For this review, take the finished solid that the model builds, in its own axes (mm). A direction names the side the tool comes from. Coordinates: 2 decimals unless noted, no trailing zeros. Loops run counter-clockwise (first coordinate to the right, second up) from the corner with the lowest first, then second, coordinate; pieces in that order, holes last. Notation, with made-up numbers: M 30.25,-38.5 L 64.25,-38.5 A25 cw 64.25,-20.5 Z; hole C -3.75,20.5 d10. An arc over 180 degrees is marked long. Answer as a JSON object with one key per item and string values. Group by question number.
Item 1: Add section A-A (x = 75). State the section outline as (y, z) points.
Item 2: Add section B-B (x = -81). State the section outline as (y, z) points.
Item 3: Wall thickness on L1, parallel to Y at x = 97.5, z = 4.35; L2, parallel to Y at x = 13.5, z = 4.9; L3, parallel to X at y = -73, z = 4.2: over which ranges is each line inside the solid? List them lowest first. Write a range as from..to.
Item 4: Insertion check: pin 1 (1.8 mm diameter, centred on x = 103.5, z = 2.5, fed in from -Y); pin 2 (3 mm diameter, centred on x = 171.5, z = 3, fed in from -Y); pin 3 (1.8 mm diameter, centred on x = -172, z = 4, fed in from +Y). Each pin has a flat end and moves straight along its axis. Give the tip position at first contact, or say it passes through.
Item 5: Mouldability with a two-part tool opening along X and no side actions: class faces 3 (the face through (3, -85, 0)), 4 (the face through (88.97, -78.69, 2.96)) as +X half, -X half, draft (parallel to the pull), parting line (faces both ways), or undercut.
Item 6: Add section C-C (z = 4.7). Count the separate pieces of the cut face and the enclosed holes in it, then the cut area to 3 significant figures.
Item 7: Tool access review of faces 1 (the face through (3, -85, 6)), 2 (the face through (-125.17, -78.85, 2.96)): name each direction out of +Z, -Z, +X, -X, +Y, -Y from which nothing blocks a thin tool from reaching the whole face with its end or side.
from build123d import *

# Parameters (mm, degrees)
SKETCH_1_R      = 1.55
SKETCH_1_R_2    = 7.9
SKETCH_1_R_3    = 1.500000002
SKETCH_1_R_4    = 1.500000001
SKETCH_1_R_5    = 1.5
SKETCH_1_R_6    = 1.25
SKETCH_1_W      = 6
SKETCH_1_H      = 10
SKETCH_1_W_2    = 10
SKETCH_1_H_2    = 6
EXTRUDE_1_DEPTH = 6


with BuildPart() as part:
    # Эскиз1 → Бобышка-Вытянуть1 (new body)
    with BuildSketch(Plane.XY):
        with BuildLine():
            Line((146.728571026, 193.302051095), (172.76481778, 193.302051095))
            ThreePointArc((172.76481778, 193.302051095), (177.038597027, 191.56796477), (178.819099243, 187.313313634))
            Line((178.819099243, 187.313313634), (178.819099243, -193.997982862))
            ThreePointArc((178.819099243, -193.997982862), (177.042504932, -198.259771734), (172.764817781, -199.997737318))
            Line((172.764817781, -199.997737318), (145.728432875, -199.997737318))
            ThreePointArc((145.728432875, -199.997737318), (142.13617765, -199.201353507), (139.217055109, -196.961432))
            Line((139.217055109, -196.961432), (136.921229056, -193.941778905))
            ThreePointArc((136.921229056, -193.941778905), (134.002106514, -191.701857397), (130.409851289, -190.905473587))
            Line((130.409851289, -190.905473587), (-129.880215727, -190.905473587))
            ThreePointArc((-129.880215727, -190.905473587), (-133.472470952, -191.701857397), (-136.391593494, -193.941778905))
            Line((-136.391593494, -193.941778905), (-138.687419547, -196.961432))
            ThreePointArc((-138.687419547, -196.961432), (-141.606542089, -199.201353507), (-145.198797314, -199.997737318))
            Line((-145.198797314, -199.997737318), (-172.235182219, -199.997737318))
            ThreePointArc((-172.235182219, -199.997737318), (-175.957867453, -198.836968562), (-178.180900757, -195.633237551))
            Line((-178.180900757, -195.633237551), (-178.180900757, 187.302262682))
            ThreePointArc((-178.180900757, 187.302262682), (-176.423541444, 191.54490337), (-172.180900757, 193.302262682))
            Line((-172.180900757, 193.302262682), (-146.198797315, 193.302262682))
            ThreePointArc((-146.198797315, 193.302262682), (-142.60654209, 194.098646493), (-139.687419548, 196.338568))
            Line((-139.687419548, 196.338568), (-136.391593495, 200.265957365))
            ThreePointArc((-136.391593495, 200.265957365), (-133.472470953, 202.505878872), (-129.880215728, 203.302262682))
            Line((-129.880215728, 203.302262682), (130.409851288, 203.302262682))
            ThreePointArc((130.409851288, 203.302262682), (134.002106513, 202.505878872), (136.921229055, 200.265957365))
            Line((136.921229055, 200.265957365), (140.217104458, 196.338462244))
            ThreePointArc((140.217104458, 196.338462244), (143.136253197, 194.098464098), (146.728571026, 193.302051095))
        make_face()
        with Locations((108.319099243, 165.602262682)):
            Circle(SKETCH_1_R, mode=Mode.SUBTRACT)
        with Locations((108.319099243, 175.302262682)):
            Circle(SKETCH_1_R, mode=Mode.SUBTRACT)
        with Locations((131.519099243, 180.302262682)):
            Circle(SKETCH_1_R_2, mode=Mode.SUBTRACT)
        with Locations((-151.980900757, 180.302262682)):
            Circle(SKETCH_1_R_2, mode=Mode.SUBTRACT)
        with Locations((-171.180900757, 150.902262682)):
            Circle(SKETCH_1_R_3, mode=Mode.SUBTRACT)
        with Locations((-171.180900757, 16.742262682)):
            Circle(SKETCH_1_R_4, mode=Mode.SUBTRACT)
        with Locations((171.819099243, 150.902051095)):
            Circle(SKETCH_1_R_4, mode=Mode.SUBTRACT)
        with Locations((126.459099243, 196.302262682)):
            Circle(SKETCH_1_R_5, mode=Mode.SUBTRACT)
        with Locations((-125.820900757, 196.302262682)):
            Circle(SKETCH_1_R_5, mode=Mode.SUBTRACT)
        with Locations((0.319099243, 196.302262682)):
            Circle(SKETCH_1_R_5, mode=Mode.SUBTRACT)
        with Locations((-119.870900757, -136.997737318)):
            Circle(SKETCH_1_R_5, mode=Mode.SUBTRACT)
        with Locations((-171.180900757, -114.967737318)):
            Circle(SKETCH_1_R_5, mode=Mode.SUBTRACT)
        with Locations((0.319099243, -136.997737318)):
            Circle(SKETCH_1_R_5, mode=Mode.SUBTRACT)
        with Locations((120.509099243, -136.997737318)):
            Circle(SKETCH_1_R_5, mode=Mode.SUBTRACT)
        with Locations((171.819099243, -114.967948905)):
            Circle(SKETCH_1_R_5, mode=Mode.SUBTRACT)
        with Locations((171.819099244, 16.742051095)):
            Circle(SKETCH_1_R_5, mode=Mode.SUBTRACT)
        with Locations((-139.980900757, 180.302262682)):
            Circle(SKETCH_1_R_6, mode=Mode.SUBTRACT)
        with Locations((-163.980900757, 180.302262682)):
            Circle(SKETCH_1_R_6, mode=Mode.SUBTRACT)
        with Locations((119.519099243, 180.302262682)):
            Circle(SKETCH_1_R_6, mode=Mode.SUBTRACT)
        with Locations((143.519099243, 180.302262682)):
            Circle(SKETCH_1_R_6, mode=Mode.SUBTRACT)
        with BuildLine():
            Line((133.65547985, 83.46981119), (133.65547985, 87.96981119))
            ThreePointArc((133.65547985, 87.96981119), (132.05547985, 89.56981119), (130.45547985, 87.96981119))
            Line((130.45547985, 87.96981119), (130.45547985, 83.46981119))
            ThreePointArc((130.45547985, 83.46981119), (132.05547985, 81.86981119), (133.65547985, 83.46981119))
        make_face(mode=Mode.SUBTRACT)
        with BuildLine():
            Line((133.65547985, 118.96981119), (133.65547985, 114.46981119))
            ThreePointArc((133.65547985, 114.46981119), (132.05547985, 112.86981119), (130.45547985, 114.46981119))
            Line((130.45547985, 114.46981119), (130.45547985, 118.96981119))
            ThreePointArc((130.45547985, 118.96981119), (132.05547985, 120.56981119), (133.65547985, 118.96981119))
        make_face(mode=Mode.SUBTRACT)
        with BuildLine():
            Line((158.55547985, 98.96981119), (158.55547985, 103.46981119))
            ThreePointArc((158.55547985, 103.46981119), (147.55547985, 114.46981119), (136.55547985, 103.46981119))
            Line((136.55547985, 103.46981119), (136.55547985, 98.96981119))
            ThreePointArc((136.55547985, 98.96981119), (147.55547985, 87.96981119), (158.55547985, 98.96981119))
        make_face(mode=Mode.SUBTRACT)
        with BuildLine():
            Line((161.45547985, 118.96981119), (161.45547985, 114.46981119))
            ThreePointArc((161.45547985, 114.46981119), (163.05547985, 112.86981119), (164.65547985, 114.46981119))
            Line((164.65547985, 114.46981119), (164.65547985, 118.96981119))
            ThreePointArc((164.65547985, 118.96981119), (163.05547985, 120.56981119), (161.45547985, 118.96981119))
        make_face(mode=Mode.SUBTRACT)
        with BuildLine():
            Line((161.45547985, 83.46981119), (161.45547985, 87.96981119))
            ThreePointArc((161.45547985, 87.96981119), (163.05547985, 89.56981119), (164.65547985, 87.96981119))
            Line((164.65547985, 87.96981119), (164.65547985, 83.46981119))
            ThreePointArc((164.65547985, 83.46981119), (163.05547985, 81.86981119), (161.45547985, 83.46981119))
        make_face(mode=Mode.SUBTRACT)
        with Locations((-171.180900756, 41.742262682)):
            Rectangle(SKETCH_1_W, SKETCH_1_H, mode=Mode.SUBTRACT)
        with Locations((94.109099243, -136.997737318)):
            Rectangle(SKETCH_1_W_2, SKETCH_1_H_2, mode=Mode.SUBTRACT)
        with Locations((146.909099243, -136.997737318)):
            Rectangle(SKETCH_1_W_2, SKETCH_1_H_2, mode=Mode.SUBTRACT)
        with Locations((-24.670900757, 196.302262682)):
            Rectangle(SKETCH_1_W_2, SKETCH_1_H_2, mode=Mode.SUBTRACT)
        with Locations((25.309099243, 196.302262682)):
            Rectangle(SKETCH_1_W_2, SKETCH_1_H_2, mode=Mode.SUBTRACT)
        with Locations((-146.270900757, -136.997737318)):
            Rectangle(SKETCH_1_W_2, SKETCH_1_H_2, mode=Mode.SUBTRACT)
        with Locations((-93.470900757, -136.997737318)):
            Rectangle(SKETCH_1_W_2, SKETCH_1_H_2, mode=Mode.SUBTRACT)
        with Locations((-25.470900757, -136.997737318)):
            Rectangle(SKETCH_1_W_2, SKETCH_1_H_2, mode=Mode.SUBTRACT)
        with Locations((26.109099243, -136.997737318)):
            Rectangle(SKETCH_1_W_2, SKETCH_1_H_2, mode=Mode.SUBTRACT)
        with Locations((-171.180900757, -8.257737318)):
            Rectangle(SKETCH_1_W, SKETCH_1_H, mode=Mode.SUBTRACT)
        with Locations((-171.180900757, 175.902262682)):
            Rectangle(SKETCH_1_W, SKETCH_1_H, mode=Mode.SUBTRACT)
        with Locations((-171.180900757, 125.902262682)):
            Rectangle(SKETCH_1_W, SKETCH_1_H, mode=Mode.SUBTRACT)
        with Locations((-171.180900756, -89.987737318)):
            Rectangle(SKETCH_1_W, SKETCH_1_H, mode=Mode.SUBTRACT)
        with Locations((-171.180900757, -139.977737318)):
            Rectangle(SKETCH_1_W, SKETCH_1_H, mode=Mode.SUBTRACT)
        with Locations((171.819099243, 41.742051095)):
            Rectangle(SKETCH_1_W, SKETCH_1_H, mode=Mode.SUBTRACT)
        with Locations((171.819099243, -8.257948905)):
            Rectangle(SKETCH_1_W, SKETCH_1_H, mode=Mode.SUBTRACT)
        with Locations((171.819099244, -89.987948905)):
            Rectangle(SKETCH_1_W, SKETCH_1_H, mode=Mode.SUBTRACT)
        with Locations((171.819099243, -139.977948905)):
            Rectangle(SKETCH_1_W, SKETCH_1_H, mode=Mode.SUBTRACT)
        Polygon((168.819099243, 170.902051095), (168.819099243, 180.902051095), (174.819099243, 180.902051095), (174.819099243, 170.978103712), (175.145177162, 170.902051095), align=None, mode=Mode.SUBTRACT)
        with Locations((171.819099243, 125.902051095)):
            Rectangle(SKETCH_1_W, SKETCH_1_H, mode=Mode.SUBTRACT)
        with Locations((-100.820900757, 196.302262682)):
            Rectangle(SKETCH_1_W_2, SKETCH_1_H_2, mode=Mode.SUBTRACT)
        with Locations((101.459099243, 196.302262682)):
            Rectangle(SKETCH_1_W_2, SKETCH_1_H_2, mode=Mode.SUBTRACT)
        with BuildLine():
            Line((-128.180900757, -71.697737318), (-128.180900757, 53.302262682))
            ThreePointArc((-128.180900757, 53.302262682), (-98.891578875, 124.012940801), (-28.180900757, 153.302262682))
            Line((-28.180900757, 153.302262682), (81.819099243, 153.302262682))
            ThreePointArc((81.819099243, 153.302262682), (88.890167055, 150.373330494), (91.819099243, 143.302262682))
            Line((91.819099243, 143.302262682), (91.819099243, -71.697737318))
            ThreePointArc((91.819099243, -71.697737318), (88.890167055, -78.768805129), (81.819099243, -81.697737318))
            Line((81.819099243, -81.697737318), (-118.180900757, -81.697737318))
            ThreePointArc((-118.180900757, -81.697737318), (-125.251968568, -78.768805129), (-128.180900757, -71.697737318))
        make_face(mode=Mode.SUBTRACT)
    extrude(amount=EXTRUDE_1_DEPTH)


solid = part.part
From the geometry:
{
 "1": {"outline": "M -190.91,0 L -81.7,0 L -81.7,6 L -190.91,6 Z; M 153.3,0 L 203.3,0 L 203.3,6 L 153.3,6 Z"},
 "2": {"outline": "M -190.91,0 L -81.7,0 L -81.7,6 L -190.91,6 Z; M 138.21,0 L 203.3,0 L 203.3,6 L 138.21,6 Z"},
 "3": {"L1": "y = -190.91..-140, -134..193.3, 199.3..203.3", "L2": "y = -190.91..-81.7, 153.3..203.3", "L3": "x = -178.18..-128.1, 91.73..178.82"},
 "4": {"pin 1": "stops at y = -190.91", "pin 2": "stops at y = -200", "pin 3": "stops at y = 193.3"},
 "5": {"face 3": "draft", "face 4": "undercut"},
 "6": {"separate pieces": "1", "enclosed holes": "48", "area": "88,700 mm²"},
 "7": {"face 1": "+Z, +X, -X, +Y, -Y", "face 2": "+Z, -Z"}
}
